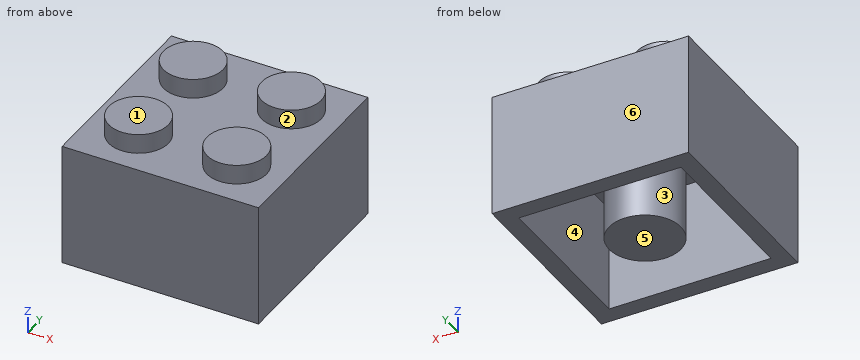
```python
from build123d import *

# Parameters (mm, degrees)
F0_W     = 16
F0_H     = 16
F1_DEPTH = 10
F2_T     = -1.4
F3_R     = 2.425
F4_DEPTH = 1.6
F5_R     = 2.925
F6_DEPTH = 10


with BuildPart() as f1:
    # F0 (on Top) → F1 (new body)
    with BuildSketch(Plane.XY):
        Rectangle(F0_W, F0_H)
    extrude(amount=F1_DEPTH)

    # F2
    f2_openings = [f1.faces().sort_by_distance(p)[0] for p in [
        (0, 0, 0),
    ]]
    offset(amount=F2_T, openings=f2_openings)

    # F3 (on face) → F4 (join)
    with BuildSketch(Plane.XY.offset(10)):
        with Locations((-4, -4)):
            Circle(F3_R)
        with Locations((-4, 4)):
            Circle(F3_R)
        with Locations((4, -4)):
            Circle(F3_R)
        with Locations((4, 4)):
            Circle(F3_R)
    extrude(amount=F4_DEPTH)

    # F5 (on face) → F6 (join)
    with BuildSketch(Plane.XY.offset(10)):
        Circle(F5_R)
    extrude(amount=-F6_DEPTH)


solid = f1.part
```
Could you check a few things on this model? Use its own coordinates, in mm. Face numbers are marked on the shaded views. A direction names the side the tool comes from. Round coordinates to 2 decimals unless told otherwise and drop trailing zeros. Loops run counter-clockwise (first coordinate to the right, second up) from the corner with the lowest first, then second, coordinate; pieces in that order, holes last. Notation, with made-up numbers: (87, 49) -> (139, 49) arc R16 ccw to (139, 79) -> close; hole circle Ø2 at (56, 11). An arc over 180 degrees is marked (long way). One line per question, with ' | ' between items.
(1) If we section it at A-A on z = 4.25: List the corners of the cut face in (x, y) for me (3 decimals), and give its area (3 significant figures).
Model answer:
outline: (-8, -8) -> (8, -8) -> (8, 8) -> (-8, 8) -> close; circle Ø5.85 at (0, 0); hole (-6.6, -6.6) -> (6.6, -6.6) -> (6.6, 6.6) -> (-6.6, 6.6) -> close | area: 109 mm^2
(2) Thinking about a two-plate mould opening in Y: for the marked faces 4, 5 and 6, which applies, released by +Y, released by -Y, zero draft, split by the parting line, or undercut?
Model answer:
face 4: undercut | face 5: zero draft | face 6: released by +Y
(3) If we section it at C-C on y = 0: List the corners of the cut face in (x, z) for me (3 decimals), and give its area (3 significant figures).
Model answer:
outline: (-8, 0) -> (-6.6, 0) -> (-6.6, 8.6) -> (-2.925, 8.6) -> (-2.925, 0) -> (2.925, 0) -> (2.925, 8.6) -> (6.6, 8.6) -> (6.6, 0) -> (8, 0) -> (8, 10) -> (-8, 10) -> close | area: 96.8 mm^2
(4) For the marked faces 1, 2 and 3, which set-ups out of +Z, -Z, +X, -X, +Y, -Y let a thin tool reach every point of the face, with its end or its side?
Model answer:
face 1: +Z, +X, -X, +Y, -Y | face 2: +Z | face 3: -Z
(5) If I drill on probe 1 along Y at (x, z) = (4.75, 6.5); probe 2 along X at (y, z) = (2, 2.25); probe 3 along X at (y, z) = (-1.75, 8.5), over which ranges is the centre line in solid material (lowest first)?
Model answer:
probe 1: y = -8 to -6.6, 6.6 to 8 | probe 2: x = -8 to -6.6, -2.13 to 2.13, 6.6 to 8 | probe 3: x = -8 to -6.6, -2.34 to 2.34, 6.6 to 8
(6) For pin 1 Ø1.5 at (x, y) = (-2, 4.5) entering from -Z, with a flat end and sliding along its axis, tell me the tip position at first contact or that it passes through.
Model answer:
pin 1: stops at z = 8.6
(7) If we section it at B-B on x = 4: List the corners of the cut face in (y, z) for me (3 decimals).
Model answer:
outline: (-8, 0) -> (-6.6, 0) -> (-6.6, 8.6) -> (6.6, 8.6) -> (6.6, 0) -> (8, 0) -> (8, 10) -> (6.425, 10) -> (6.425, 11.6) -> (1.575, 11.6) -> (1.575, 10) -> (-1.575, 10) -> (-1.575, 11.6) -> (-6.425, 11.6) -> (-6.425, 10) -> (-8, 10) -> close
